from build123d import *

# Parameters (mm, degrees)
CROQUIS1_W              = 35
CROQUIS1_H              = 58
SALIENTE_EXTRUIR1_DEPTH = 18
CROQUIS2_R              = 6.171851971
SALIENTE_EXTRUIR2_DEPTH = 16
REDONDEO1_R             = 5
REDONDEO2_R             = 1
CROQUIS3_R              = 2.99773064
CROQUIS3_R_2            = 2.835456682
CORTAR_EXTRUIR1_DEPTH   = 16
CROQUIS4_W              = 12.151773781
CROQUIS4_H              = 16.202365041
CROQUIS4_H_2            = 14.488653354
SALIENTE_EXTRUIR3_DEPTH = 2


with BuildPart() as part:
    # Croquis1 → Saliente-Extruir1 (new body)
    with BuildSketch(Plane.XY):
        Rectangle(CROQUIS1_W, CROQUIS1_H)
    extrude(amount=SALIENTE_EXTRUIR1_DEPTH)

    # Croquis2 → Saliente-Extruir2 (add)
    with BuildSketch(Plane.ZY.offset(17.5)):
        with Locations(Location((8, -21.714410647, 0), (0, 0, 90))):
            Circle(CROQUIS2_R)
    extrude(amount=SALIENTE_EXTRUIR2_DEPTH)

    # Redondeo1
    redondeo1_edges = [part.edges().sort_by_distance(p)[0] for p in [
        (17.5, -29, 9),
        (17.5, 29, 9),
    ]]
    fillet(redondeo1_edges, radius=REDONDEO1_R)

    # Redondeo2
    redondeo2_edges = [part.edges().sort_by_distance(p)[0] for p in [
        (-2.5, -29, 18),
        (17.5, 0, 0),
        (17.5, 0, 18),
        (-2.5, 29, 0),
        (16.035533906, 27.535533906, 0),
        (16.035533906, -27.535533906, 0),
        (-2.5, 29, 18),
        (16.035533906, 27.535533906, 18),
        (16.035533906, -27.535533906, 18),
        (-2.5, -29, 0),
    ]]
    fillet(redondeo2_edges, radius=REDONDEO2_R)

    # Croquis3 → Cortar-Extruir1 (cut)
    with BuildSketch(Plane.XY.offset(18)):
        with Locations((-13.764302947, 23.174055768)):
            Circle(CROQUIS3_R)
        with Locations((-13.764302947, -20.681384223)):
            Circle(CROQUIS3_R_2)
    extrude(amount=-CORTAR_EXTRUIR1_DEPTH, mode=Mode.SUBTRACT)

    # Croquis4 → Saliente-Extruir3 (add)
    with BuildSketch(Plane(origin=(17.5, 0, 0), x_dir=(0, 0, -1), z_dir=(1, 0, 0))):
        with Locations((-9.467375914, 11.333865931)):
            Rectangle(CROQUIS4_W, CROQUIS4_H)
        with Locations((-9.467375914, -10.087530158)):
            Rectangle(CROQUIS4_W, CROQUIS4_H_2)
    extrude(amount=SALIENTE_EXTRUIR3_DEPTH)


solid = part.part
The listing builds one solid part. Answer for the finished solid, in the listing's coordinates (mm). A direction names the side the tool comes from. Round coordinates to 2 decimals unless told otherwise and drop trailing zeros. Order: outer loops, then holes, each group sorted by start corner. A loop starts at its lowest first (then second) coordinate and runs counter-clockwise, first axis right, second up. Notation, with made-up numbers: M 56,86 L 62,86 A32 ccw 62,120 Z; hole C 49.25,36.25 d3. An arc over 180 degrees is marked long. Answer in a Markdown table with one row per item. Add a question column.
1) Flat-ended cylindrical pins translate along their axes: pin 1 Ø9 at (y, z) = (2, 9) entering from -X; pin 2 Ø0.6 at (x, z) = (18.5, 7) entering from -Y; pin 3 Ø1.6 at (x, z) = (18.5, 9.5) entering from +Y. Find the tip coordinate at first contact, or state that the pin passes through.
2) The part is cut by section A-A on y = 7. Determine the outline of the cut face in (x, z).
3) Which of the six approach directions +Z, -Z, +X, -X, +Y, -Y give full straight-line access (tool end or side, diameter ignored) to faces 1 (the face through (18, -10, 15.543)), 2 (the face through (18, -17.332, 10)), 3 (the face through (-14, -21, 2))?
4) Consider line 1 along Y through (x, z) = (-14, 5.25); line 2 along X through (y, z) = (-14, 8.25); line 3 along X through (y, z) = (21, 6). Determine where each line is inside the solid, lowest interval first. Write a range as from..to.
5) Determine the mould class of faces 4 (the face through (-3, -29, 9)), 5 (the face through (-15.974, 25.2, 10.112)), 6 (the face through (-33.5, -22, 8)) for opening direction Y: pulls with the +Y half, pulls with the -Y half, needs draft (parallel to the pull), parting line crosses it, or undercut.
6) The part is cut by section B-B on z = 6.5. Determine the outline of the cut face in (x, y).
7) The part is cut by section C-C on x = -15.5. Determine the outline of the cut face in (y, z).
8) The part is cut by section D-D on x = -29. Determine the outline of the cut face in (y, z), plus the area to 3 significant figures.
Findings below:
| question | item | result |
|---|---|---|
| 1 | pin 1 | stops at x = -17.5 |
| 1 | pin 2 | stops at y = -17.33 |
| 1 | pin 3 | stops at y = 19.44 |
| 2 | outline | M -17.5,0 L 16.5,0 A1 ccw 17.5,1 L 17.5,3.39 L 19.5,3.39 L 19.5,15.54 L 17.5,15.54 L 17.5,17 A1 ccw 16.5,18 L -17.5,18 Z |
| 3 | face 1 | +Z, +X, +Y, -Y |
| 3 | face 2 | +Z, -Z, +X, -Y |
| 3 | face 3 | +Z |
| 4 | line 1 | y = -29..-23.51, -17.86..20.19, 26.16..29 |
| 4 | line 2 | x = -17.5..19.5 |
| 4 | line 3 | x = -17.5..-15.83, -11.7..17.5 |
| 5 | face 4 | pulls with the -Y half |
| 5 | face 5 | undercut |
| 5 | face 6 | needs draft |
| 6 | outline | M -33.5,-27.7 L -17.5,-27.7 L -17.5,-29 L 12.5,-29 A5 ccw 17.5,-24 L 17.5,-17.33 L 19.5,-17.33 L 19.5,-2.84 L 17.5,-2.84 L 17.5,3.23 L 19.5,3.23 L 19.5,19.44 L 17.5,19.44 L 17.5,24 A5 ccw 12.5,29 L -17.5,29 L -17.5,-15.73 L -33.5,-15.73 Z; hole C -13.76,23.17 d6; hole C -13.76,-20.68 d5.67 |
| 7 | outline | M -29,1 A1 ccw -28,0 L 28,0 A1 ccw 29,1 L 29,17 A1 ccw 28,18 L 25.62,18 L 25.62,2 L 20.73,2 L 20.73,18 L -18.44,18 L -18.44,2 L -22.92,2 L -22.92,18 L -28,18 A1 ccw -29,17 Z |
| 8 | outline | C -21.71,8 d12.34 |
| 8 | area | 120 mm² |
